The drawing under review shows one solid part. Ordinate dimensions are in mm from its lowest x, y, z. Round coordinates to 2 decimals unless told otherwise and drop trailing zeros. Order: outer loops, then holes, each group sorted by start corner. A loop starts at its lowest first (then second) coordinate and runs counter-clockwise, first axis right, second up. Notation, with made-up numbers: M 24,23 L 75,23 A23 cw 75,58 Z; hole C 30.5,-11 d8. An arc over 180 degrees is marked long. Answer as a JSON object with one key per item and string values. Group by question number.
1. Add section B-B on z = 745.5. State the section outline as (x, y) points, and give its area (3 significant figures).
2. Add section A-A on x = 97. State the section outline as (y, z) points.
3. Clearance check with flat-ended pins moving along their axes: P1, Ø7.5, axis at x = 524.5, y = 16.5, coming from the -Z side; P2, Ø12.5, axis at y = 14.5, z = 2252.5, coming from the -X side. State where each tip first meets the part, or that it passes through.
4. To check wall thickness, follow probe 1 along Z at (x, y) = (408, 21); probe 2 along X at (y, z) = (9.5, 1242). State the ranges of each line that lie inside material, in increasing order. Write a range as [from, to].
5. Add section C-C on y = 13. State the section outline as (x, z) points, and give its area (3 significant figures).
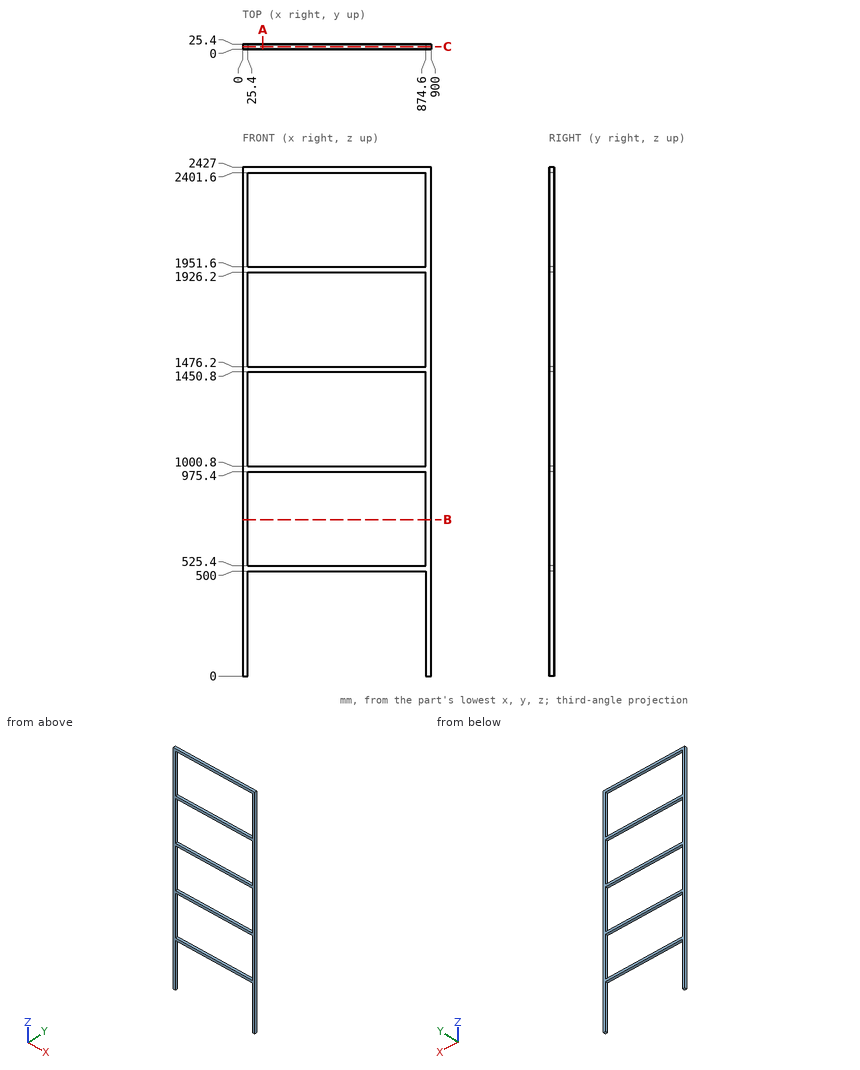
Recorded:
{
 "1": {"outline": "M 0,0 L 25.4,0 L 25.4,25.4 L 0,25.4 Z; M 874.6,0 L 900,0 L 900,25.4 L 874.6,25.4 Z", "area": "1,290 mm²"},
 "2": {"outline": "M 0,500 L 25.4,500 L 25.4,525.4 L 0,525.4 Z; M 0,975.4 L 25.4,975.4 L 25.4,1000.8 L 0,1000.8 Z; M 0,1450.8 L 25.4,1450.8 L 25.4,1476.2 L 0,1476.2 Z; M 0,1926.2 L 25.4,1926.2 L 25.4,1951.6 L 0,1951.6 Z; M 0,2401.6 L 25.4,2401.6 L 25.4,2427 L 0,2427 Z"},
 "3": {"P1": "stops at z = 500", "P2": "stops at x = 0"},
 "4": {"probe 1": "z = [500, 525.4], [975.4, 1000.8], [1450.8, 1476.2], [1926.2, 1951.6], [2401.6, 2427]", "probe 2": "x = [0, 25.4], [874.6, 900]"},
 "5": {"outline": "M 0,0 L 25.4,0 L 25.4,500 L 874.6,500 L 874.6,0 L 900,0 L 900,2427 L 0,2427 Z; hole M 25.4,525.4 L 874.6,525.4 L 874.6,975.4 L 25.4,975.4 Z; hole M 25.4,1000.8 L 874.6,1000.8 L 874.6,1450.8 L 25.4,1450.8 Z; hole M 25.4,1476.2 L 874.6,1476.2 L 874.6,1926.2 L 25.4,1926.2 Z; hole M 25.4,1951.6 L 874.6,1951.6 L 874.6,2401.6 L 25.4,2401.6 Z", "area": "231,000 mm²"}
}
